from build123d import *

# Parameters (mm, degrees)
BOSS_EXTRUDE1_DEPTH = 2.5
FILLET1_R           = 0.5
FILLET2_R           = 1


with BuildPart() as part:
    # Sketch1 → Boss-Extrude1 (new body)
    with BuildSketch(Plane.XY):
        with BuildLine():
            Line((0, 4), (8.614511907, 5.991904768))
            ThreePointArc((8.614511907, 5.991904768), (16.104194038, -0.749209679), (7.206608675, -5.479002182))
            Line((7.206608675, -5.479002182), (8.001476125, -3.91993652))
            ThreePointArc((8.001476125, -3.91993652), (12.64885164, 3.513343848), (6.781304612, -3))
            Line((6.781304612, -3), (5.708406149, -4))
            Line((5.708406149, -4), (0, -2))
            Line((0, -2), (0, 4))
        make_face()
    boss_extrude1 = extrude(amount=BOSS_EXTRUDE1_DEPTH)

    # Mirror1: Boss-Extrude1 across plane
    add(boss_extrude1.mirror(Plane(origin=(0, 4, 2.5), x_dir=(0, 0, 1), z_dir=(1, 0, 0))))

    # Fillet1
    fillet1_edges = [part.edges().sort_by_distance(p)[0] for p in [
        (7.206608675, -5.479002182, 1.25),
        (-7.206608675, -5.479002182, 1.25),
    ]]
    fillet(fillet1_edges, radius=FILLET1_R)

    # Fillet2
    fillet2_edges = [part.edges().sort_by_distance(p)[0] for p in [
        (6.781304612, -3, 1.25),
        (-6.781304612, -3, 1.25),
    ]]
    fillet(fillet2_edges, radius=FILLET2_R)


solid = part.part
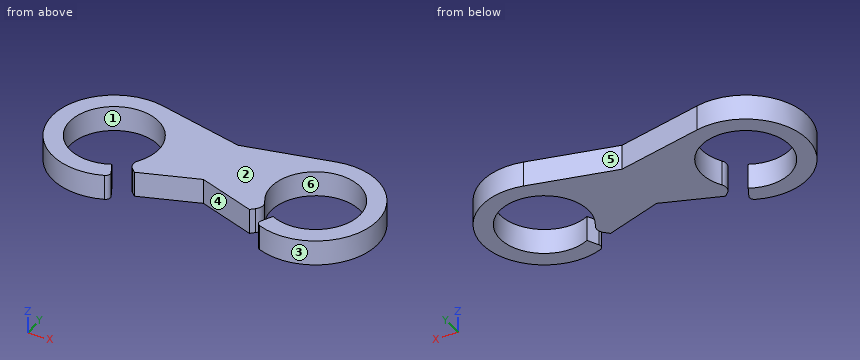
The model under review builds one solid part; all positions refer to its coordinate system, in mm. Face numbers are marked on the shaded views. A direction names the side the tool comes from. Coordinates: 2 decimals unless noted, no trailing zeros. Write each loop counter-clockwise with the first axis right and the second up, starting at its lowest first coordinate (ties: lowest second). Pieces come first, ordered by that corner, then holes. Notation, with made-up numbers: M -23.5,22 L 26.5,22 A24 cw 26.5,38 Z; hole C 79.5,76 d4. An arc over 180 degrees is marked long. Put each result on its own line as item: value.
1) Wall thickness on probe 1 along X at (y, z) = (0.25, 1.55); probe 2 along Y at (x, z) = (10, 1.35); probe 3 along X at (y, z) = (1.75, 0.45): over which ranges is each line inside the solid? List them lowest first. Write a range as [from, to].
Computed:
probe 1: x = [-16.14, -14.39], [-5.61, 5.61], [14.39, 16.14]
probe 2: y = [-6.15, -4.4], [4.4, 6.15]
probe 3: x = [-15.9, -14.04], [-5.96, 5.96], [14.04, 15.9]
2) Add section D-D on z = 1.55. Give the boundary of the cut face in (x, y).
Computed:
outline: M -8.61,5.99 A6.15 ccw long -7.7,-5.7 A0.5 ccw -7.44,-5.01 L -8,-3.92 A4.4 cw long -6.28,-2.35 A1 ccw -6.12,-3.62 L -5.71,-4 L 0,-2 L 5.71,-4 L 6.12,-3.62 A1 ccw 6.28,-2.35 A4.4 cw long 8,-3.92 L 7.44,-5.01 A0.5 ccw 7.7,-5.7 A6.15 ccw long 8.61,5.99 L 0,4 Z
3) Add section A-A on y = 0. Give the boundary of the cut face in (x, z).
Computed:
outline: M -16.15,0 L -14.4,0 L -14.4,2.5 L -16.15,2.5 Z; M -5.6,0 L 5.6,0 L 5.6,2.5 L -5.6,2.5 Z; M 14.4,0 L 16.15,0 L 16.15,2.5 L 14.4,2.5 Z
4) Add section C-C on y = 5. Give the boundary of the cut face in (x, z).
Computed:
outline: M -13.58,0 L -4.32,0 L -4.32,2.5 L -13.58,2.5 Z; M 4.32,0 L 13.58,0 L 13.58,2.5 L 4.32,2.5 Z
5) Clearance check with a flat-ended pin moving along its axis: pin 1 Ø1 at (y, z) = (2.5, 1.5) entering from +X. State where the tip first meets the part, or that it passes through.
Computed:
pin 1: stops at x = 15.82
6) Draft analysis for pull direction Y (two halves, no side actions). For the marked faces 1, 2 and 3, state which applies: released by +Y, released by -Y, zero draft, split by the parting line, or undercut.
Computed:
face 1: undercut
face 2: zero draft
face 3: split by the parting line
7) For the marked faces 4, 5 and 6, list the 3-axis set-ups (+Z, -Z, +X, -X, +Y, -Y) from which the entire face can be reached by the end or side of a thin tool; tool diameter is ignored.
Computed:
face 4: +Z, -Z, -Y
face 5: +Z, -Z, +Y
face 6: +Z, -Z
8) Add section B-B on x = -10. Give the boundary of the cut face in (y, z), then the cut area to 3 significant figures.
Computed:
outline: M -6.15,0 L -4.4,0 L -4.4,2.5 L -6.15,2.5 Z; M 4.4,0 L 6.15,0 L 6.15,2.5 L 4.4,2.5 Z
area: 8.75 mm2
